Input: part model. Units: mm. Frame: model coordinates. A direction names the side the tool comes from. Round coordinates to 2 decimals unless told otherwise and drop trailing zeros. Loops run counter-clockwise (first coordinate to the right, second up) from the corner with the lowest first, then second, coordinate; pieces in that order, holes last. Notation, with made-up numbers: M 71,3.5 L 120,3.5 A19 cw 120,19.5 Z; hole C 68.25,35.5 d7. An arc over 180 degrees is marked long. Return JSON: item names as keys, results as strings. Group by question number.
1) Section A-A (x = -115.5). Output: boundary loops of the cut face in (y, z), plus the area to 3 significant figures.
2) Access query for faces 4 (the face through (-3, -74, 32)), 5 (the face through (79, -73, 17)), 6 (the face through (115, 3, -3.5)), 7 (the face through (-17, -74, 9)), 8 (the face through (16, -74, 19)). Directions: +Z, -Z, +X, -X, +Y, -Y. A direction counts if a zero-diameter tool reaches every point of the face in a straight line with its end or side. Return the directions, or none.
3) Section D-D (z = 14). Output: boundary loops of the cut face in (x, y), plus the area to 3 significant figures.
4) Section B-B (y = 48.5). Output: boundary loops of the cut face in (x, z).
5) Contact query for flat-ended pins moving along their axis: P1, Ø4, axis at y = -73.5, z = 16, coming from the +X side; P2, Ø3, axis at x = 115.5, y = 57.5, coming from the -Z side; P3, Ø12, axis at y = -10, z = 13.5, coming from the -X side; P4, Ø12, axis at x = -55, y = -39.5, coming from the -Z side. Output: stop coordinate, or through.
6) Mould query, pull axis X, two halves, no side actions, for faces 1 (the face through (-49, -74, 28)), 2 (the face through (37, -74, 32)), 3 (the face through (-84, -74, 19)). Classes: +X half, -X half, draft (parallel to the pull), parting line (faces both ways), or undercut.
7) Material intervals for line 1 (Y direction, x = -115.5, z = -4.8); line 2 (Y direction, x = -115, z = -4); line 3 (X direction, y = 57, z = -4), sorted ascending. Write a range as from..to.
8) Section C-C (y = -57.5). Output: boundary loops of the cut face in (x, z), plus the area to 3 significant figures.
from build123d import *

# Parameters (mm, degrees)
F0_W      = 198
F0_H      = 135
F1_DEPTH  = 37
F3_DEPTH  = 135
F4_R      = 2.5
F5_DEPTH  = 25
F7_DEPTH  = 7
F9_DEPTH  = 13
F10_W     = 11
F10_H     = 11
F11_DEPTH = 12


with BuildPart() as f1:
    # F0 (on Top) → F1 (new body)
    with BuildSketch(Plane.XY):
        Rectangle(F0_W, F0_H)
    extrude(amount=F1_DEPTH)

    # F2 (on face) → F3 (join, through all)
    with BuildSketch(Plane.XZ.offset(67.5)):
        Polygon((-108.5, -3.5), (-122.5, -3.5), (-122.5, -5.5), (-107.933711, -5.5), (-99, 0), (-99, 2.348633), align=None)
        Polygon((99, 2.348633), (99, 0), (107.933711, -5.5), (122.5, -5.5), (122.5, -3.5), (108.5, -3.5), align=None)
    extrude(amount=-F3_DEPTH)

    # F4 (on face) → F5 (cut)
    with BuildSketch(Plane(origin=(0, 0, -5.5), x_dir=(1, 0, 0), z_dir=(0, 0, -1))):
        with Locations((-115.5, 57.5)):
            Circle(F4_R)
        with Locations((-115.5, -57.5)):
            Circle(F4_R)
        with Locations((115.5, -57.5)):
            Circle(F4_R)
        with Locations((115.5, 57.5)):
            Circle(F4_R)
    extrude(amount=-F5_DEPTH, mode=Mode.SUBTRACT)

    # F6 (on face) → F7 (join)
    with BuildSketch(Plane(origin=(0, 67.5, 0), x_dir=(-1, 0, 0), z_dir=(0, 1, 0))):
        Polygon((-122.5, -5.5), (-107.933711, -5.5), (-99, 0), (99, 0), (107.933711, -5.5), (122.5, -5.5), (122.5, -3.5), (108.5, -3.5), (99, 2.348633), (-99, 2.348633), (-108.5, -3.5), (-122.5, -3.5), align=None)
    extrude(amount=F7_DEPTH)

    # F8 (on face) → F9 (join)
    with BuildSketch(Plane.XZ.offset(67.5)):
        Polygon((-77.5, 28), (-84, 28), (-84, 9), (-82, 9), (-82, 6), (-59, 6), (-59, 9), (-57, 9), (-57, 28), (-63.5, 28), (-63.5, 32), (-77.5, 32), align=None)
        Polygon((-45, 28), (-54, 28), (-54, 9), (-49.5, 9), (-49.5, 6), (-26.5, 6), (-26.5, 9), (-22, 9), (-22, 28), (-31, 28), (-31, 32), (-45, 32), align=None)
        Polygon((-10, 28), (-19, 28), (-19, 9), (-14.5, 9), (-14.5, 6), (8.5, 6), (8.5, 9), (13, 9), (13, 28), (4, 28), (4, 32), (-10, 32), align=None)
        Polygon((30, 28), (16, 28), (16, 9), (25.5, 9), (25.5, 6), (48.5, 6), (48.5, 9), (58, 9), (58, 28), (44, 28), (44, 32), (30, 32), align=None)
    extrude(amount=F9_DEPTH)

    # F10 (on face) → F11 (join)
    with BuildSketch(Plane.XZ.offset(67.5)):
        with Locations((79.5, 11.5)):
            Rectangle(F10_W, F10_H)
    extrude(amount=F11_DEPTH)


solid = f1.part
Returned:
{
 "1": {"outline": "M -67.5,-5.5 L -60,-5.5 L -60,-3.5 L -67.5,-3.5 Z; M -55,-5.5 L 55,-5.5 L 55,-3.5 L -55,-3.5 Z; M 60,-5.5 L 74.5,-5.5 L 74.5,-3.5 L 60,-3.5 Z", "area": "264 mm^2"},
 "2": {"face 4": "+Z, +X, -X, -Y", "face 5": "+Z, +X, -Y", "face 6": "+Z, +X, +Y, -Y", "face 7": "-Z, -Y", "face 8": "+Z, -Z, -Y"},
 "3": {"outline": "M -99,-67.5 L -84,-67.5 L -84,-80.5 L -57,-80.5 L -57,-67.5 L -54,-67.5 L -54,-80.5 L -22,-80.5 L -22,-67.5 L -19,-67.5 L -19,-80.5 L 13,-80.5 L 13,-67.5 L 16,-67.5 L 16,-80.5 L 58,-80.5 L 58,-67.5 L 74,-67.5 L 74,-79.5 L 85,-79.5 L 85,-67.5 L 99,-67.5 L 99,67.5 L -99,67.5 Z", "area": "28,600 mm^2"},
 "4": {"outline": "M -122.5,-5.5 L -107.93,-5.5 L -99,0 L 99,0 L 107.93,-5.5 L 122.5,-5.5 L 122.5,-3.5 L 108.5,-3.5 L 99,2.35 L 99,37 L -99,37 L -99,2.35 L -108.5,-3.5 L -122.5,-3.5 Z"},
 "5": {"P1": "stops at x = 85", "P2": "passes through", "P3": "stops at x = -99", "P4": "stops at z = 0"},
 "6": {"face 1": "undercut", "face 2": "draft", "face 3": "-X half"},
 "7": {"line 1": "y = -67.5..-60, -55..55, 60..74.5", "line 2": "y = -67.5..-59.95, -55.05..55.05, 59.95..74.5", "line 3": "x = -122.5..-117.95, -113.05..-105.5, 105.5..113.05, 117.95..122.5"},
 "8": {"outline": "M -122.5,-5.5 L -118,-5.5 L -118,-3.5 L -122.5,-3.5 Z; M -113,-5.5 L -107.93,-5.5 L -99,0 L 99,0 L 107.93,-5.5 L 113,-5.5 L 113,-3.5 L 108.5,-3.5 L 99,2.35 L 99,37 L -99,37 L -99,2.35 L -108.5,-3.5 L -113,-3.5 Z; M 118,-5.5 L 122.5,-5.5 L 122.5,-3.5 L 118,-3.5 Z", "area": "7,410 mm^2"}
}
